Input: dimensioned drawing with shaded views. Units: mm. Origin: part minimum x, y, z. A direction names the side the tool comes from. Give positions to 0.01 mm unless a question says otherwise; leave off trailing zeros. Write each loop counter-clockwise with the first axis right and the second up, starting at its lowest first coordinate (ties: lowest second). Pieces come first, ordered by that corner, then holes. Notation, with made-up numbers: M -28.75,40.25 L 2.25,40.25 A14 cw 2.25,60.25 Z; hole C 84.5,51 d8. An arc over 180 degrees is marked long. Use CSV: the item, a comma, the result in double quotes. Start each with the question number.
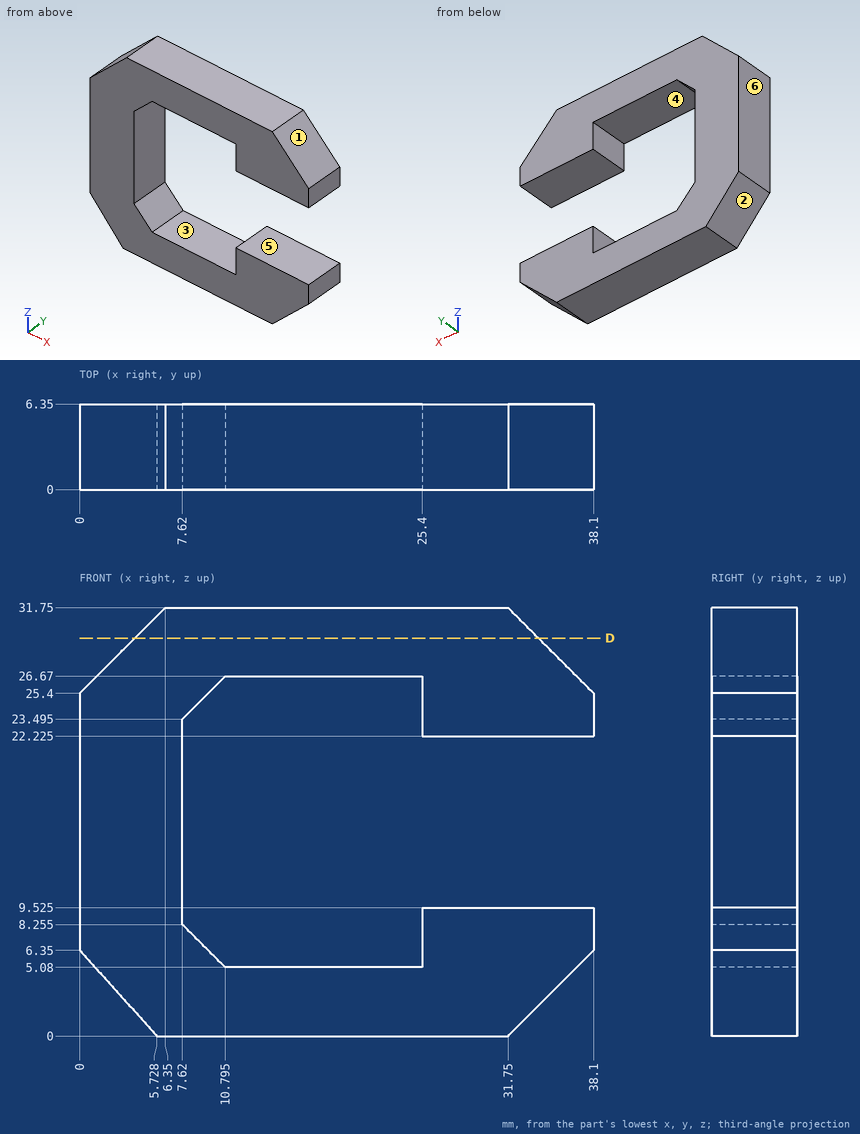
Item 1: Pull-direction query (X, two-part tool) for the marked faces 1, 2 and 3; classes: released by +X, released by -X, zero draft, split by the parting line, or undercut.
Item 2: Set-up query: the marked faces 4, 5 and 6. Return all of +Z, -Z, +X, -X, +Y, -Y with unobstructed straight access to the full face (end or side cutting, diameter ignored); none if empty.
Item 3: Section D-D (z = 29.5). Return the cut outline in (x, y).
Item 4: Contact query for flat-ended pins moving along their axis: pin 1 Ø1.9 at (x, y) = (31.5, 2.5) entering from -Z; pin 2 Ø3 at (y, z) = (3, 15) entering from +X. Output: stop coordinate, or through.
Item 5: Material intervals for probe 1 along Z at (x, y) = (19, 4.25); probe 2 along X at (y, z) = (0.75, 9); probe 3 along X at (y, z) = (3.25, 17), sorted ascending.
Output values:
1,face 1,"released by +X"
1,face 2,"released by -X"
1,face 3,"undercut"
2,face 4,"+Y, -Y"
2,face 5,"+X, +Y, -Y"
2,face 6,"+Z, -Z, -X, +Y, -Y"
3,outline,"M 4.1,0 L 34,0 L 34,6.35 L 4.1,6.35 Z"
4,pin 1,"stops at z = 0"
4,pin 2,"stops at x = 7.62"
5,probe 1,"z = 0 to 5.08, 26.67 to 31.75"
5,probe 2,"x = 0 to 7.62, 25.4 to 38.1"
5,probe 3,"x = 0 to 7.62"
